Drawing for the job (mm, zero at the part's lowest x, y, z). A direction names the side the tool comes from. Round coordinates to 2 decimals unless told otherwise and drop trailing zeros. Write each loop counter-clockwise with the first axis right and the second up, starting at its lowest first coordinate (ties: lowest second). Pieces come first, ordered by that corner, then holes. Notation, with made-up numbers: M 81.25,53 L 85.25,53 A25 cw 85.25,77 Z; hole C 81,-39 d2. An arc over 180 degrees is marked long. Use a Markdown table: item, result.
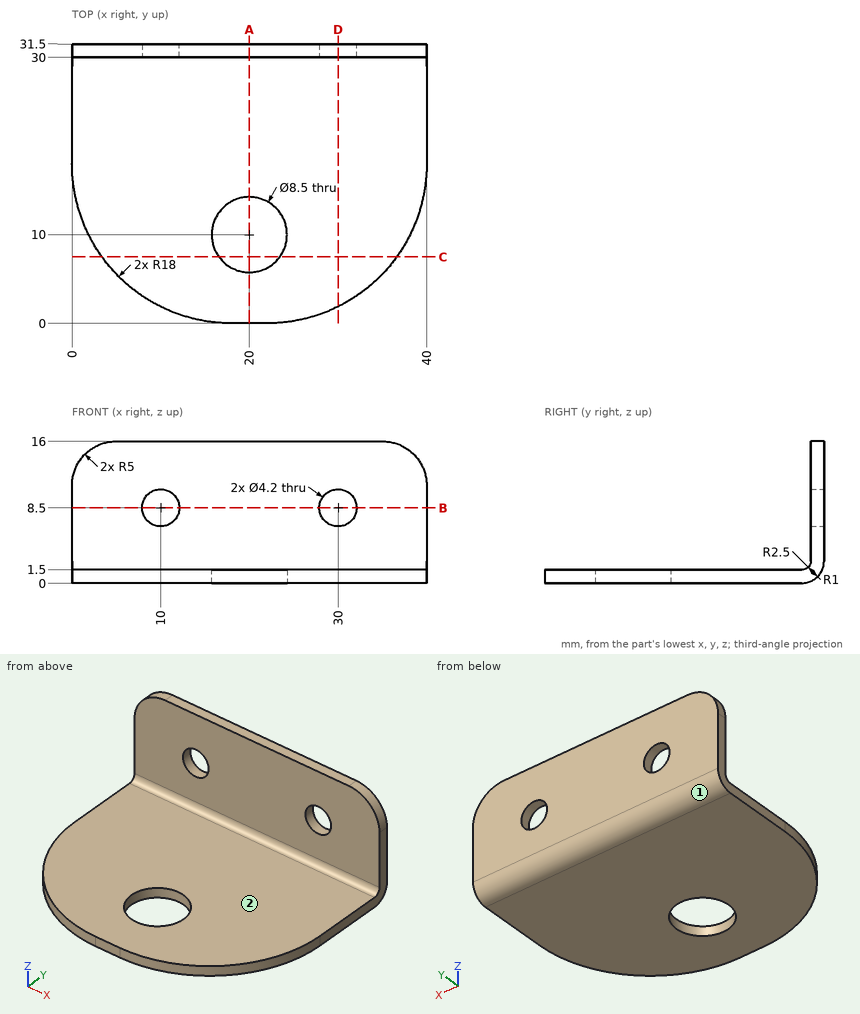
Q1. Cut at B-B on z = 8.5. Give the cut face in (x, y), and give its area (3 significant figures).
Response values:
| item | result |
|---|---|
| outline | M 0,30 L 7.9,30 L 7.9,31.5 L 0,31.5 Z; M 12.1,30 L 27.9,30 L 27.9,31.5 L 12.1,31.5 Z; M 32.1,30 L 40,30 L 40,31.5 L 32.1,31.5 Z |
| area | 47.4 mm2 |
Q2. Which spindle directions (+Z, -Z, +X, -X, +Y, -Y) get a long thin tool onto all of the face, cutting with end or side? Do the marked faces 1 and 2. Say none if no direction does.
Response values:
| item | result |
|---|---|
| face 1 | -Z, +X, -X, +Y |
| face 2 | +Z, +X, -X, -Y |
Q3. Cut at A-A on x = 20. Give the cut face in (y, z), and give its area (3 significant figures).
Response values:
| item | result |
|---|---|
| outline | M 0,0 L 5.75,0 L 5.75,1.5 L 0,1.5 Z; M 14.25,0 L 29,0 A2.5 ccw 31.5,2.5 L 31.5,16 L 30,16 L 30,2.5 A1 cw 29,1.5 L 14.25,1.5 Z |
| area | 55.1 mm2 |
Q4. Drill centre lines: L1, parallel to Z at x = 11, y = 11.5; L2, parallel to Y at x = 24.5, z = 14.5; L3, parallel to Z at x = 10, y = 30.9. Where is each one in solid material? Low to high.
Response values:
| item | result |
|---|---|
| L1 | z = 0 to 1.5 |
| L2 | y = 30 to 31.5 |
| L3 | z = 0.88 to 6.4, 10.6 to 16 |
Q5. Cut at D-D on x = 30. Give the cut face in (y, z), and give its area (3 significant figures).
Response values:
| item | result |
|---|---|
| outline | M 1.88,0 L 29,0 A2.5 ccw 31.5,2.5 L 31.5,6.4 L 30,6.4 L 30,2.5 A1 cw 29,1.5 L 1.88,1.5 Z; M 30,10.6 L 31.5,10.6 L 31.5,16 L 30,16 Z |
| area | 58.8 mm2 |
Q6. Cut at C-C on y = 7.5. Give the cut face in (x, z).
Response values:
| item | result |
|---|---|
| outline | M 3.38,0 L 16.56,0 L 16.56,1.5 L 3.38,1.5 Z; M 23.44,0 L 36.62,0 L 36.62,1.5 L 23.44,1.5 Z |
Q7. Drop flat-ended pins along their axis: P1, Ø11, axis at x = 20, y = 10, coming from the +Z side; P2, Ø2, axis at x = 19, z = 13.5, coming from the -Y side. Give the stop position or say it passes through.
Response values:
| item | result |
|---|---|
| P1 | stops at z = 1.5 |
| P2 | stops at y = 30 |
